Work out the finished part from the listing and answer in its coordinate system (mm). Give positions to 0.01 mm unless a question says otherwise; leave off trailing zeros. Loops run counter-clockwise (first coordinate to the right, second up) from the corner with the lowest first, then second, coordinate; pieces in that order, holes last. Notation, with made-up numbers: (31, 0) - (57, 0) arc R31 cw to (57, 32) - close; hole circle Ø11 at (-1.5, 1.25). An arc over 180 degrees is marked (long way). One line per question, with ' | ' between items. Start each with the question number.
1. Find the intervals of material crossed by line 1 (Z direction, x = 2.45, y = 42); line 2 (X direction, y = 19, z = -22); line 3 (Z direction, x = 3.7, y = 6), in increasing order.
2. Section A-A (x = 2.5) is taken. Determine the outline of the cut face in (y, z).
3. Section B-B (z = -3) is taken. Determine the outline of the cut face in (x, y), plus the area to 3 significant figures.
4. For a pull along Z with two mould halves and no side action, classify faces 1 (the face through (3, 0, -18)), 2 (the face through (1, 22, -35)), 3 (the face through (3.17, 22.185, -4.617)) as released by +Z, released by -Z, zero draft, split by the parting line, or undercut.
5. Section C-C (y = 31) is taken. Determine the outline of the cut face in (x, z), plus the area to 3 significant figures.
6. This flat-tipped pin is pushed along its axis until it touches: pin 1 (1.5 mm diameter, centred on x = 3.5, y = 20.5, fed in from +Z). Where does it stop, or does it pass through?
from build123d import *

# Parameters (mm, degrees)
SKETCH1_R           = 1.75
BOSS_EXTRUDE1_DEPTH = 45


with BuildPart() as part:
    # Sketch1 → Boss-Extrude1 (new body)
    with BuildSketch(Plane(origin=(0, 0, 0), x_dir=(1, 0, 0), z_dir=(0, 1, 0))):
        with BuildLine():
            Line((0, 35), (3, 35))
            ThreePointArc((3, 35), (4.414213562, 34.414213562), (5, 33))
            Line((5, 33), (5, 2))
            ThreePointArc((5, 2), (4.414213562, 0.585786438), (3, 0))
            Line((3, 0), (0, 0))
            Line((0, 0), (0, 35))
        make_face()
        with Locations(Location((2.5, 32, 0), (0, 0, 90))):
            Circle(SKETCH1_R, mode=Mode.SUBTRACT)
        with Locations(Location((2.5, 22, 0), (0, 0, 90))):
            Circle(SKETCH1_R, mode=Mode.SUBTRACT)
        with Locations(Location((2.5, 13, 0), (0, 0, 90))):
            Circle(SKETCH1_R, mode=Mode.SUBTRACT)
        with Locations(Location((2.5, 3, 0), (0, 0, 90))):
            Circle(SKETCH1_R, mode=Mode.SUBTRACT)
    extrude(amount=BOSS_EXTRUDE1_DEPTH)


solid = part.part
Conclusion:
1) line 1: -35 to -33.75, -30.25 to -23.75, -20.25 to -14.75, -11.25 to -4.75, -1.25 to 0 | line 2: 0 to 0.75, 4.25 to 5 | line 3: -34.87 to -33.27, -30.73 to -23.27, -20.73 to -14.27, -11.73 to -4.27, -1.73 to -0.13
2) outline: (0, -35) - (45, -35) - (45, -33.75) - (0, -33.75) - close; (0, -30.25) - (45, -30.25) - (45, -23.75) - (0, -23.75) - close; (0, -20.25) - (45, -20.25) - (45, -14.75) - (0, -14.75) - close; (0, -11.25) - (45, -11.25) - (45, -4.75) - (0, -4.75) - close; (0, -1.25) - (45, -1.25) - (45, 0) - (0, 0) - close
3) outline: (0, 0) - (0.75, 0) - (0.75, 45) - (0, 45) - close; (4.25, 0) - (5, 0) - (5, 45) - (4.25, 45) - close | area: 67.5 mm²
4) face 1: zero draft | face 2: released by -Z | face 3: undercut
5) outline: (0, -35) - (3, -35) arc R2 ccw to (5, -33) - (5, -2) arc R2 ccw to (3, 0) - (0, 0) - close; hole circle Ø3.5 at (2.5, -32); hole circle Ø3.5 at (2.5, -22); hole circle Ø3.5 at (2.5, -13); hole circle Ø3.5 at (2.5, -3) | area: 135 mm²
6) pin 1: z = 0
